Part model, mm, in its own coordinate system. A direction names the side the tool comes from. Round coordinates to 2 decimals unless told otherwise and drop trailing zeros. Answer as a JSON object with one key per item and string values. Group by question number.
1. Drop flat-ended pins along their axis: pin 1 (5 mm diameter, centred on x = 13, y = 0.5, fed in from +Z); pin 2 (0.5 mm diameter, centred on x = -24.5, y = 11.5, fed in from +Z). Give the stop position or say it passes through.
2. Two-plate mould, pull along X, no slides. Class faces 3 (the face through (0, 12.7, -1)), 4 (the face through (-25.4, 0, -1)), 5 (the face through (25.4, 0, -1)), 6 (the face through (25, -12, -0.914)): +X half, -X half, draft (parallel to the pull), parting line (faces both ways), or undercut.
3. Which spindle directions (+Z, -Z, +X, -X, +Y, -Y) get a long thin tool onto all of the face, cutting with end or side? Do faces 1 (the face through (-25, -12, -0.914)), 2 (the face through (0, 0, 0)). Say none if no direction does.
from build123d import *

# Parameters (mm, degrees)
SKETCH1_W           = 50.8
SKETCH1_H           = 25.4
BOSS_EXTRUDE1_DEPTH = 1.778
SKETCH2_R           = 0.762
CUT_EXTRUDE2_DEPTH  = 0.9144


with BuildPart() as part:
    # Sketch1 → Boss-Extrude1 (new body)
    with BuildSketch(Plane.XY):
        Rectangle(SKETCH1_W, SKETCH1_H)
    extrude(amount=-BOSS_EXTRUDE1_DEPTH)

    # Sketch2 → Cut-Extrude2 (cut)
    with BuildSketch(Plane.XY):
        with Locations((-24.511, 11.811)):
            Circle(SKETCH2_R)
        with Locations(Location((24.511, 11.811, 0), (0, 0, 180))):
            Circle(SKETCH2_R)
        with Locations((24.511, -11.811)):
            Circle(SKETCH2_R)
        with Locations(Location((-24.511, -11.811, 0), (0, 0, 180))):
            Circle(SKETCH2_R)
    extrude(amount=-CUT_EXTRUDE2_DEPTH, mode=Mode.SUBTRACT)


solid = part.part
Worked answers:
{
 "1": {"pin 1": "stops at z = 0", "pin 2": "stops at z = -0.91"},
 "2": {"face 3": "draft", "face 4": "-X half", "face 5": "+X half", "face 6": "undercut"},
 "3": {"face 1": "+Z", "face 2": "+Z, +X, -X, +Y, -Y"}
}
